from build123d import *

# Parameters (mm, degrees)
SKETCH1_W           = 24
SKETCH1_H           = 21
SKETCH1_R           = 1.625
BOSS_EXTRUDE1_DEPTH = 8
SKETCH2_W           = 50
SKETCH2_H           = 34
SKETCH2_R           = 1.625
BOSS_EXTRUDE2_DEPTH = 2
FILLET2_R           = 2.5
SKETCH3_W           = 50
SKETCH3_H           = 2.861592732
BOSS_EXTRUDE3_DEPTH = 10
SKETCH4_R           = 2.5625
CUT_EXTRUDE3_DEPTH  = 3


with BuildPart() as part:
    # Sketch1 → Boss-Extrude1 (new body)
    with BuildSketch(Plane(origin=(0, 0, 0), x_dir=(1, 0, 0), z_dir=(0, 1, 0))):
        Rectangle(SKETCH1_W, SKETCH1_H)
        with Locations(Location((-9.5, 8, 0), (0, 0, 270))):
            Circle(SKETCH1_R, mode=Mode.SUBTRACT)
        with Locations(Location((9.5, 8, 0), (0, 0, 270))):
            Circle(SKETCH1_R, mode=Mode.SUBTRACT)
        with Locations(Location((9.5, -8, 0), (0, 0, 270))):
            Circle(SKETCH1_R, mode=Mode.SUBTRACT)
        with Locations(Location((-9.5, -8, 0), (0, 0, 270))):
            Circle(SKETCH1_R, mode=Mode.SUBTRACT)
    extrude(amount=BOSS_EXTRUDE1_DEPTH)

    # Sketch2 → Boss-Extrude2 (add)
    with BuildSketch(Plane(origin=(0, 8, 0), x_dir=(1, 0, 0), z_dir=(0, 1, 0))):
        with Locations((-13, 0)):
            Rectangle(SKETCH2_W, SKETCH2_H)
        with Locations(Location((9.5, -8, 0), (0, 0, 270))):
            Circle(SKETCH2_R, mode=Mode.SUBTRACT)
        with Locations(Location((-9.5, -8, 0), (0, 0, 270))):
            Circle(SKETCH2_R, mode=Mode.SUBTRACT)
        with Locations(Location((9.5, 8, 0), (0, 0, 270))):
            Circle(SKETCH2_R, mode=Mode.SUBTRACT)
        with Locations(Location((-9.5, 8, 0), (0, 0, 270))):
            Circle(SKETCH2_R, mode=Mode.SUBTRACT)
    extrude(amount=BOSS_EXTRUDE2_DEPTH)

    # Fillet2
    fillet2_edges = [part.edges().sort_by_distance(p)[0] for p in [
        (0, 8, -10.5),
        (-12, 8, 0),
        (0, 8, 10.5),
    ]]
    fillet(fillet2_edges, radius=FILLET2_R)

    # Sketch3 → Boss-Extrude3 (add)
    with BuildSketch(Plane(origin=(0, 10, 0), x_dir=(1, 0, 0), z_dir=(0, 1, 0))):
        with Locations((-13, 15.569203634)):
            Rectangle(SKETCH3_W, SKETCH3_H)
        with Locations((-13, -15.569203634)):
            Rectangle(SKETCH3_W, SKETCH3_H)
    extrude(amount=BOSS_EXTRUDE3_DEPTH)

    # Sketch4 → Cut-Extrude3 (cut)
    with BuildSketch(Plane(origin=(0, 10, 0), x_dir=(1, 0, 0), z_dir=(0, 1, 0))):
        with Locations(Location((-9.5, 8, 0), (0, 0, 270))):
            Circle(SKETCH4_R)
        with Locations((9.5, 8)):
            Circle(SKETCH4_R)
        with Locations((9.5, -8)):
            Circle(SKETCH4_R)
        with Locations(Location((-9.5, -8, 0), (0, 0, 270))):
            Circle(SKETCH4_R)
    extrude(amount=-CUT_EXTRUDE3_DEPTH, mode=Mode.SUBTRACT)


solid = part.part
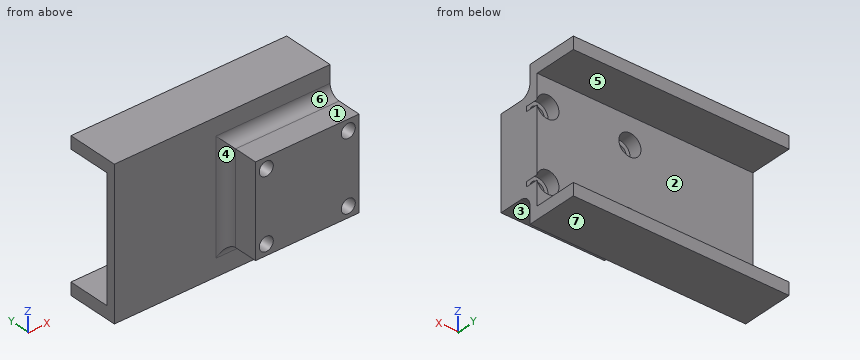
The listing builds one solid part. Answer for the finished solid, in the listing's coordinates (mm). Face numbers are marked on the shaded views. A direction names the side the tool comes from. Coordinates: 2 decimals unless noted, no trailing zeros. Write each loop counter-clockwise with the first axis right and the second up, starting at its lowest first coordinate (ties: lowest second). Pieces come first, ordered by that corner, then holes. Notation, with made-up numbers: M -6,65.5 L 52,65.5 A30 cw 52,96.5 Z; hole C -4,-31 d11. An arc over 180 degrees is marked long. Use one line per item in the form item = value.
Item 1: Find section D-D, the plane y = 4.5. Give the vertices of the cut face in (x, z) (3 decimals), plus the area to 3 significant figures.
Model answer:
outline = M -12,-10.5 L 12,-10.5 L 12,10.5 L -12,10.5 Z; hole C -9.5,-8 d3.25; hole C -9.5,8 d3.25; hole C 9.5,-8 d3.25; hole C 9.5,8 d3.25
area = 471 mm2
Item 2: Given P1, Ø10, axis at x = -17.5, z = -3.5, coming from the -Y side; P2, Ø4, axis at x = -9.5, z = -8, coming from the +Y side; P3, Ø6, axis at x = -9.5, z = 8, coming from the +Y side, each flat-ended and moving along its own axis, determine where each tip first touches the part or whether it passes through.
Model answer:
P1 = 7
P2 = 7
P3 = 10
Item 3: Find the intervals of material crossed by probe 1 along X at (y, z) = (4.5, -8) (3 decimals); probe 2 along Z at (x, y) = (9.5, 8.5); probe 3 along Z at (x, y) = (9.5, 5.75) (3 decimals), in increasing order.
Model answer:
probe_1 = -12 to -11.125, -7.875 to 7.875, 11.125 to 12
probe_2 = -17 to -10.56, -5.44 to 5.44, 10.56 to 17
probe_3 = -10.513 to -9.625, -6.375 to 6.375, 9.625 to 10.513
Item 4: Find section B-B, the plane z = -8. Give the vertices of the cut face in (x, y) (1 decimal).
Model answer:
outline = M -38,8 L -14.5,8 A2.5 cw -12,5.5 L -12,0 L -11.1,0 L -11.1,7 L -12.1,7 L -12.1,10 L -38,10 Z; M -7.9,0 L 7.9,0 L 7.9,7 L 6.9,7 L 6.9,10 L -6.9,10 L -6.9,7 L -7.9,7 Z; M 11.1,0 L 12,0 L 12,7 L 11.1,7 Z
Item 5: For the marked faces 1, 2 and 3, determine the directions among +Z, -Z, +X, -X, +Y, -Y from which every point of the face is accessible in a straight line to the end or side of a thin tool.
Model answer:
face_1 = +Z, +X, -X, -Y
face_2 = +X, -X, +Y
face_3 = -Z, +X, -X, -Y
Item 6: The mould has two halves that part along Z. Classify the marked faces 4, 5, 6 and 7: released by +Z, released by -Z, zero draft, split by the parting line, or undercut.
Model answer:
face_4 = zero draft
face_5 = undercut
face_6 = released by +Z
face_7 = released by -Z
Item 7: Find section A-A, the plane y = 11. Give the vertices of the cut face in (x, z), plus the area to 3 significant figures.
Model answer:
outline = M -38,-17 L 12,-17 L 12,-14.14 L -38,-14.14 Z; M -38,14.14 L 12,14.14 L 12,17 L -38,17 Z
area = 286 mm2
Item 8: Find section C-C, the plane x = 9.5. Give the number of separate pieces and of enclosed holes in the cut face, plus the area to 3 significant figures.
Model answer:
separate_pieces = 3
enclosed_holes = 0
area = 220 mm2
